```python
from build123d import *

# Parameters (mm, degrees)
SKETCH1_W           = 50
SKETCH1_H           = 90
SKETCH1_R           = 3
BOSS_EXTRUDE1_DEPTH = 20
SKETCH2_R           = 3.35
CUT_EXTRUDE1_DEPTH  = 156.32224567
CUT_EXTRUDE2_DEPTH  = 159.271917913
CHAMFER1_SIZE       = 3


with BuildPart() as part:
    # Sketch1 → Boss-Extrude1 (new body)
    with BuildSketch(Plane.XY):
        with Locations((100, 50)):
            Rectangle(SKETCH1_W, SKETCH1_H)
        with Locations((115, 20)):
            Circle(SKETCH1_R, mode=Mode.SUBTRACT)
        with Locations((85, 20)):
            Circle(SKETCH1_R, mode=Mode.SUBTRACT)
        with Locations((85, 50)):
            Circle(SKETCH1_R, mode=Mode.SUBTRACT)
        with Locations((115, 50)):
            Circle(SKETCH1_R, mode=Mode.SUBTRACT)
    extrude(amount=BOSS_EXTRUDE1_DEPTH)

    # Sketch2 → Cut-Extrude1 (cut, through all)
    with BuildSketch(Plane(origin=(0, 95, 0), x_dir=(1, 0, 0), z_dir=(0, 1, 0))):
        with Locations(Location((100, -7.5, 0), (0, 0, 270))):
            Circle(SKETCH2_R)
    extrude(amount=-CUT_EXTRUDE1_DEPTH, mode=Mode.SUBTRACT)

    # Sketch3 → Cut-Extrude2 (cut, through all)
    with BuildSketch(Plane.XY.offset(20)):
        Polygon((90, 70), (90, 74), (110, 74), (110, 70), (110, 30), (90, 30), align=None)
    extrude(amount=-CUT_EXTRUDE2_DEPTH, mode=Mode.SUBTRACT)

    # Chamfer1
    chamfer1_edges = [part.edges().sort_by_distance(p)[0] for p in [
        (75, 50, 20),
        (100, 5, 20),
        (125, 50, 20),
        (100, 95, 20),
    ]]
    chamfer(chamfer1_edges, length=CHAMFER1_SIZE)


solid = part.part
```
Input: part model. Units: mm. Frame: model coordinates. A direction names the side the tool comes from. Round coordinates to 2 decimals unless told otherwise and drop trailing zeros. Loops run counter-clockwise (first coordinate to the right, second up) from the corner with the lowest first, then second, coordinate; pieces in that order, holes last. Notation, with made-up numbers: (72, 4.25) - (100, 4.25) arc R7 ccw to (100, 9.25) - close; hole circle Ø4 at (47, 38.25). An arc over 180 degrees is marked (long way). One line per item, written item: value. Start each with the question number.
(1) Section C-C, the plane z = 2.5. Return loops of the section in (x, y).
(2) Contact query for flat-ended pins moving along their axis: P1, Ø5, axis at x = 85, y = 50, coming from the -Z side; P2, Ø10, axis at x = 88.5, y = 56.5, coming from the -Z side. Output: stop coordinate, or through.
(3) Ray query, line 1 (Y direction, x = 85, z = 11.25); line 2 (X direction, y = 85.5, z = 7.5); line 3 (Y direction, x = 103, z = 2.5). Return the intervals inside material, ascending. Write a range as [from, to].
(4) Section A-A, the plane y = 20. Return loops of the section in (x, z), plus the area to 3 significant figures.
(5) Access query for faces 5 (the flat face through (100, 74, 12)), 6 (the flat face through (125, 49, 8)). Directions: +Z, -Z, +X, -X, +Y, -Y. A direction counts if a zero-diameter tool reaches every point of the face in a straight line with its end or side. Return the directions, or none.
(6) Section D-D, the plane x = 100. Return loops of the section in (y, z), plus the area to 3 significant figures.
(7) Draft query along X for faces 1 (the flat face through (124, 49, 18)), 2 (the flat face through (100, 93, 19)), 3 (the flat face through (90, 52, 10)), 4 (the flat face through (75, 49, 8)). Return one class per face: +X half, -X half, draft (parallel to the pull), parting line (faces both ways), or undercut.
(8) Section B-B, the plane x = 85. Return loops of the section in (y, z), plus the area to 3 significant figures.
Results below:
1. outline: (75, 5) - (125, 5) - (125, 95) - (75, 95) - close; hole circle Ø6 at (85, 20); hole circle Ø6 at (85, 50); hole (90, 30) - (110, 30) - (110, 74) - (90, 74) - close; hole circle Ø6 at (115, 20); hole circle Ø6 at (115, 50)
2. P1: through
2. P2: z = 0
3. line 1: [5, 17], [23, 47], [53, 95]
3. line 2: [75, 96.65], [103.35, 125]
3. line 3: [5, 30], [74, 95]
4. outline: (75, 0) - (82, 0) - (82, 20) - (78, 20) - (75, 17) - close; (88, 0) - (112, 0) - (112, 20) - (88, 20) - close; (118, 0) - (125, 0) - (125, 17) - (122, 20) - (118, 20) - close; hole circle Ø6.7 at (100, 7.5)
4. area: 716 mm^2
5. face 5: +Z, -Z
5. face 6: +Z, -Z, +X, +Y, -Y
6. outline: (5, 0) - (30, 0) - (30, 4.15) - (5, 4.15) - close; (5, 10.85) - (30, 10.85) - (30, 20) - (8, 20) - (5, 17) - close; (74, 0) - (95, 0) - (95, 4.15) - (74, 4.15) - close; (74, 10.85) - (95, 10.85) - (95, 17) - (92, 20) - (74, 20) - close
6. area: 603 mm^2
7. face 1: +X half
7. face 2: draft
7. face 3: undercut
7. face 4: -X half
8. outline: (5, 0) - (17, 0) - (17, 20) - (8, 20) - (5, 17) - close; (23, 0) - (47, 0) - (47, 20) - (23, 20) - close; (53, 0) - (95, 0) - (95, 17) - (92, 20) - (53, 20) - close
8. area: 1,550 mm^2
